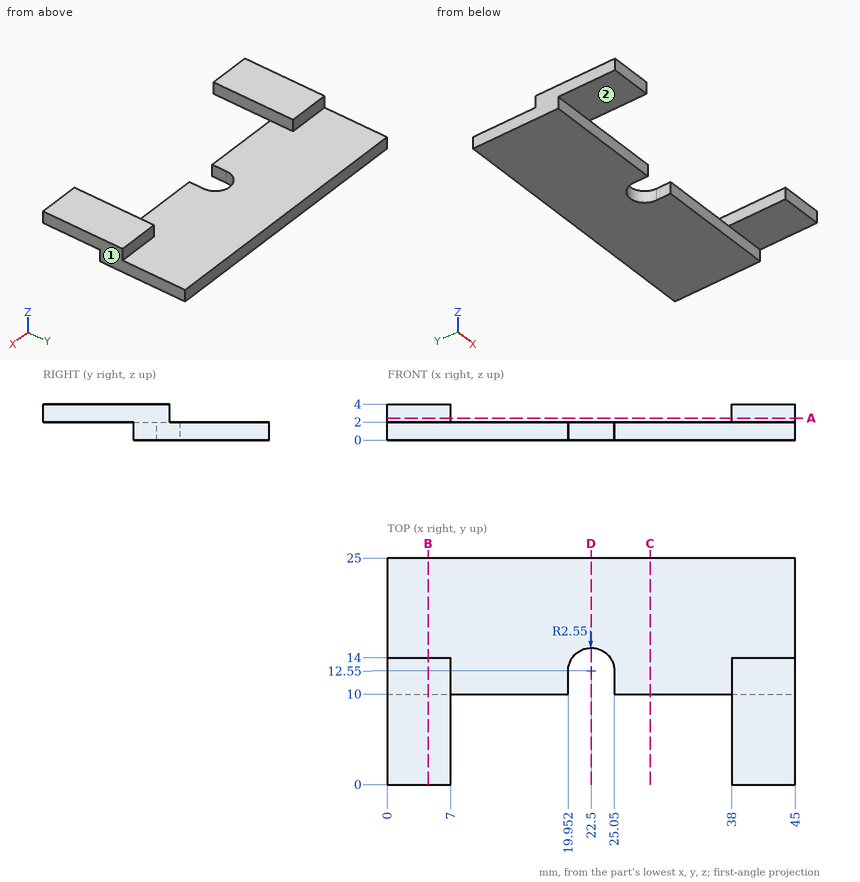
Drawing for the job (mm, zero at the part's lowest x, y, z). A direction names the side the tool comes from. Give positions to 0.01 mm unless a question says otherwise; leave off trailing zeros. Order: outer loops, then holes, each group sorted by start corner. A loop starts at its lowest first (then second) coordinate and runs counter-clockwise, first axis right, second up. Notation, with made-up numbers: (54.5, 81.5) - (94.5, 81.5) arc R11 cw to (94.5, 102.5) - close; hole circle Ø7 at (-12, 52). An arc over 180 degrees is marked (long way). Write item = value, one per line. Start each with the question number.
1. Cut at B-B, the plane x = 4.5. List the corners of the cut face in (y, z).
2. Drop flat-ended pins along their axis: P1, Ø1.6, axis at x = 4.5, z = 3, coming from the +Y side; P2, Ø7.5, axis at x = 2, y = 3.5, coming from the -Z side; P3, Ø0.6, axis at y = 11, z = 1, coming from the -X side; P4, Ø0.6, axis at x = 38, z = 0.5, coming from the -Y side. Give the stop position or say it passes through.
3. Which spindle directions (+Z, -Z, +X, -X, +Y, -Y) get a long thin tool onto all of the face, cutting with end or side? Do the marked faces 1 and 2. Say none if no direction does.
4. Cut at A-A, the plane z = 2.45. List the corners of the cut face in (x, y).
5. Cut at D-D, the plane x = 22.5. List the corners of the cut face in (y, z).
6. Probe line 1 along Y through (x, z) = (5, 2.25); line 2 along X through (y, z) = (10.75, 2.9); line 3 along Z through (x, y) = (4, 2.5). List the from-to ranges inside material, lowest first.
7. Cut at C-C, the plane x = 29. List the corners of the cut face in (y, z), and give its area (3 significant figures).
Taken from the geometry:
q1.outline = (0, 2) - (10, 2) - (10, 0) - (25, 0) - (25, 2) - (14, 2) - (14, 4) - (0, 4) - close
q2.P1 = 14
q2.P2 = 2
q2.P3 = 0
q2.P4 = 10
q3.face_1 = +Z, -Z, +X, +Y, -Y
q3.face_2 = -Z, +X, -X, -Y
q4.outline = (0, 0) - (7, 0) - (7, 14) - (0, 14) - close; (38, 0) - (45, 0) - (45, 14) - (38, 14) - close
q5.outline = (15.1, 0) - (25, 0) - (25, 2) - (15.1, 2) - close
q6.line_1 = 0 to 14
q6.line_2 = 0 to 7, 38 to 45
q6.line_3 = 2 to 4
q7.outline = (10, 0) - (25, 0) - (25, 2) - (10, 2) - close
q7.area = 30.0 mm²
